Geometry: final body of the model. Coordinates: model frame, mm. Face numbers are marked on the shaded views. A direction names the side the tool comes from. Give positions to 0.01 mm unless a question says otherwise; leave off trailing zeros. Use CSV: the item, a comma, the result in double quotes.
```python
from build123d import *

# Parameters (mm, degrees)
SKETCH2_R           = 60.96
BOSS_EXTRUDE1_DEPTH = 3.556
FILLET1_R           = 0.762
SKETCH3_W           = 128.524
SKETCH3_H           = 12.7
BOSS_EXTRUDE2_DEPTH = 3.556
SKETCH4_W           = 12.7
SKETCH4_H           = 128.524
BOSS_EXTRUDE3_DEPTH = 3.556
FILLET2_R           = 0.762
SKETCH3_2_W         = 128.524
SKETCH3_2_H         = 12.7
BOSS_EXTRUDE4_DEPTH = 3.556
SKETCH4_2_W         = 12.7
SKETCH4_2_H         = 128.524
BOSS_EXTRUDE5_DEPTH = 3.556


with BuildPart() as part:
    # Sketch2 → Boss-Extrude1 (new body)
    with BuildSketch(Plane.XY):
        Circle(SKETCH2_R)
    extrude(amount=BOSS_EXTRUDE1_DEPTH)

    # Fillet1
    fillet1_edges = [part.edges().sort_by_distance(p)[0] for p in [
        (-60.96, 0, 0),
        (-60.96, 0, 3.556),
    ]]
    fillet(fillet1_edges, radius=FILLET1_R)

    # Sketch3 → Boss-Extrude2 (add)
    with BuildSketch(Plane.XY):
        Rectangle(SKETCH3_W, SKETCH3_H)
    extrude(amount=-BOSS_EXTRUDE2_DEPTH)

    # Sketch4 → Boss-Extrude3 (add)
    with BuildSketch(Plane.XY):
        Rectangle(SKETCH4_W, SKETCH4_H)
    extrude(amount=-BOSS_EXTRUDE3_DEPTH)

    # Fillet2
    fillet2_edges = [part.edges().sort_by_distance(p)[0] for p in [
        (35.306, 6.35, -3.556),
        (-64.262, 6.35, -1.778),
        (64.262, 0, -3.556),
        (64.262, 6.35, -1.778),
        (-35.306, -6.35, -3.556),
        (64.262, -6.35, -1.778),
        (-64.262, 0, -3.556),
        (-64.262, -6.35, -1.778),
        (-35.306, 6.35, -3.556),
        (35.306, -6.35, -3.556),
        (6.35, 35.306, -3.556),
        (6.35, 64.262, -1.778),
        (-6.35, 35.306, -3.556),
        (6.35, -35.306, -3.556),
        (0, -64.262, -3.556),
        (6.35, -64.262, -1.778),
        (-6.35, -35.306, -3.556),
        (-6.35, -64.262, -1.778),
        (0, 64.262, -3.556),
        (-6.35, 64.262, -1.778),
    ]]
    fillet(fillet2_edges, radius=FILLET2_R)

    # Sketch3<2> → Boss-Extrude4 (add)
    with BuildSketch(Plane.XY):
        Rectangle(SKETCH3_2_W, SKETCH3_2_H)
    extrude(amount=BOSS_EXTRUDE4_DEPTH)

    # Sketch4<2> → Boss-Extrude5 (add)
    with BuildSketch(Plane.XY):
        Rectangle(SKETCH4_2_W, SKETCH4_2_H)
    extrude(amount=BOSS_EXTRUDE5_DEPTH)


solid = part.part
```
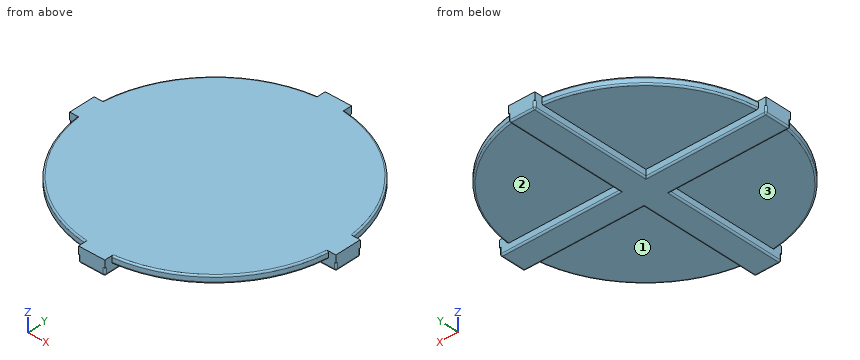
1. Line query: line 1 (X direction, y = 32.5, z = -2.5); line 2 (Z direction, x = 23.5, y = -32); line 3 (X direction, y = 5, z = -3). Output: solid intervals per line, ascending.
Answer:
line 1,"-6.35 to 6.35"
line 2,"0 to 3.56"
line 3,"-64.23 to 64.23"
2. Reachability of the marked faces 1, 2 and 3 from +Z, -Z, +X, -X, +Y, -Y: full face, straight path, thin tool, end or side. Return the list, or none.
Answer:
face 1,"-Z, +X, -Y"
face 2,"-Z, +X, +Y"
face 3,"-Z, -X, -Y"
3. Pin query (flat end, axial travel): pin 1 Ø1.9 at (x, z) = (47, -1) entering from -Y; pin 2 Ø3 at (x, z) = (-34.5, -0.5) entering from -Y; pin 3 Ø4 at (x, y) = (39, 35) entering from -Z. Return the tip coordinate at first contact, or that it passes through.
Answer:
pin 1,"y = -6.35"
pin 2,"y = -50.96"
pin 3,"z = 0"
